The listing builds one solid part. Answer for the finished solid, in the listing's coordinates (mm). Face numbers are marked on the shaded views. A direction names the side the tool comes from. Coordinates: 2 decimals unless noted, no trailing zeros. Order: outer loops, then holes, each group sorted by start corner. A loop starts at its lowest first (then second) coordinate and runs counter-clockwise, first axis right, second up.
```python
from build123d import *

# Parameters (mm, degrees)
SKETCH1_W            = 68.5
SKETCH1_H            = 64.5
BOSS_EXTRUDE3_DEPTH  = 19
SKETCH3_W            = 60.5
SKETCH3_H            = 60.5
CUT_EXTRUDE1_DEPTH   = 15
SKETCH5_W            = 68.5
SKETCH5_H            = 4
BOSS_EXTRUDE4_DEPTH  = 105
SKETCH10_W           = 10
SKETCH10_H           = 29
BOSS_EXTRUDE5_DEPTH  = 5.5
SKETCH9_W            = 4
SKETCH9_H            = 20
CUT_EXTRUDE2_DEPTH   = 20.5
SKETCH11_W           = 6
SKETCH11_H           = 20
CUT_EXTRUDE3_DEPTH   = 5.5
CHAMFER2_SIZE        = 5.5
CHAMFER3_SIZE        = 2
SKETCH12_W           = 34.25
SKETCH12_H           = 169.5
CUT_EXTRUDE4_DEPTH   = 50
SKETCH15_R           = 1.5
CUT_EXTRUDE5_DEPTH   = 50
SKETCH16_R           = 1.5
CUT_EXTRUDE6_DEPTH   = 50
SKETCH17_R           = 1.5
CUT_EXTRUDE7_DEPTH   = 50
SKETCH19_W           = 34.25
SKETCH19_H           = 4
BOSS_EXTRUDE6_DEPTH  = 2
SKETCH26_W           = 4
SKETCH26_H           = 4
BOSS_EXTRUDE7_DEPTH  = 30
SKETCH20_R           = 3.75
CUT_EXTRUDE9_DEPTH   = 179.453250181
SKETCH21_W           = 3
SKETCH21_H           = 2.563068229
CUT_EXTRUDE10_DEPTH  = 5
SKETCH18_R           = 1.5
CUT_EXTRUDE8_DEPTH   = 135
SKETCH24_R           = 4
CUT_EXTRUDE13_DEPTH  = 178.441011325
SKETCH25_W           = 3
SKETCH25_H           = 2.291900756
CUT_EXTRUDE14_DEPTH  = 5
SKETCH27_R           = 1.75
CUT_EXTRUDE15_DEPTH  = 178.441011325
BOSS_EXTRUDE9_START  = 5
SKETCH30_W           = 8
SKETCH30_H           = 8
SKETCH30_R           = 1.75
BOSS_EXTRUDE9_DEPTH  = 5
SKETCH31_W           = 8
SKETCH31_H           = 8
CUT_EXTRUDE16_DEPTH  = 5
SKETCH32_W           = 19.705511252
SKETCH32_H           = 17.257631466
BOSS_EXTRUDE10_DEPTH = 5
SKETCH33_R           = 1.5
CUT_EXTRUDE17_DEPTH  = 5
SKETCH34_R           = 3.75
CUT_EXTRUDE18_DEPTH  = 5
SKETCH35_W           = 3
SKETCH35_H           = 2.563068229
CUT_EXTRUDE19_DEPTH  = 5


# Some blends are built 0.0001 mm under size
with BuildPart() as part:
    # Sketch1 → Boss-Extrude3 (new body)
    with BuildSketch(Plane(origin=(0, 0, 0), x_dir=(1, 0, 0), z_dir=(0, 1, 0))):
        with Locations((-34.25, 32.25)):
            Rectangle(SKETCH1_W, SKETCH1_H)
    extrude(amount=BOSS_EXTRUDE3_DEPTH)

    # Sketch3 → Cut-Extrude1 (cut)
    with BuildSketch(Plane(origin=(0, 19, 0), x_dir=(1, 0, 0), z_dir=(0, 1, 0))):
        with Locations((-34.25, 34.25)):
            Rectangle(SKETCH3_W, SKETCH3_H)
    extrude(amount=-CUT_EXTRUDE1_DEPTH, mode=Mode.SUBTRACT)

    # Sketch5 → Boss-Extrude4 (add)
    with BuildSketch(Plane(origin=(0, 0, -64.5), x_dir=(-1, 0, 0), z_dir=(0, 0, -1))):
        with Locations((34.25, 2)):
            Rectangle(SKETCH5_W, SKETCH5_H)
    extrude(amount=BOSS_EXTRUDE4_DEPTH)

    # Sketch10 → Boss-Extrude5 (add)
    with BuildSketch(Plane.XZ):
        with Locations((-5, -30)):
            Rectangle(SKETCH10_W, SKETCH10_H)
    extrude(amount=BOSS_EXTRUDE5_DEPTH)

    # Sketch9 → Cut-Extrude2 (cut)
    with BuildSketch(Plane(origin=(0, 19, 0), x_dir=(1, 0, 0), z_dir=(0, 1, 0))):
        with Locations((-2, 28)):
            Rectangle(SKETCH9_W, SKETCH9_H)
    extrude(amount=-CUT_EXTRUDE2_DEPTH, mode=Mode.SUBTRACT)

    # Sketch11 → Cut-Extrude3 (cut)
    with BuildSketch(Plane(origin=(0, 4, 0), x_dir=(1, 0, 0), z_dir=(0, 1, 0))):
        with Locations((-7, 28)):
            Rectangle(SKETCH11_W, SKETCH11_H)
    extrude(amount=-CUT_EXTRUDE3_DEPTH, mode=Mode.SUBTRACT)

    # Chamfer2
    chamfer2_edges = [part.edges().sort_by_distance(p)[0] for p in [
        (-5, -5.5, -44.5),
        (-5, -5.5, -15.5),
    ]]
    chamfer(chamfer2_edges, length=CHAMFER2_SIZE - 0.0001)  # a hair under: the kernel refuses the full size

    # Chamfer3
    # the kernel refuses this chamfer: 2 mm, written as the material it adds along each edge
    with BuildSketch(Plane(origin=(0, -1.5, -38), x_dir=(0, 0.9996219169112968, -0.027495876610585623), z_dir=(-1, 0, 0)), Plane(origin=(0, -1.5, -18), x_dir=(0, -0.027495876610586403, -0.9996219169112968), z_dir=(-1, 0, 0))) as chamfer3_piece_1:
        Polygon((CHAMFER3_SIZE * 0.999621916911, -CHAMFER3_SIZE * 0.0274958766106), (-CHAMFER3_SIZE * 0.0274958766106, -CHAMFER3_SIZE * 0.999621916911), (0, 0), align=None)
    extrude(amount=10)

    # Sketch12 → Cut-Extrude4 (cut)
    with BuildSketch(Plane(origin=(0, 19, 0), x_dir=(1, 0, 0), z_dir=(0, 1, 0))):
        with Locations((-51.375, 84.75)):
            Rectangle(SKETCH12_W, SKETCH12_H)
    extrude(amount=-CUT_EXTRUDE4_DEPTH, mode=Mode.SUBTRACT)

    # Sketch15 → Cut-Extrude5 (cut)
    with BuildSketch(Plane(origin=(0, -1.5, 0), x_dir=(1, 0, 0), z_dir=(0, 1, 0))):
        with Locations(Location((-5, 31.75713966, 0), (0, 0, 270))):
            Circle(SKETCH15_R)
    extrude(amount=-CUT_EXTRUDE5_DEPTH, mode=Mode.SUBTRACT)

    # Sketch16 → Cut-Extrude6 (cut)
    with BuildSketch(Plane(origin=(0, 4, 0), x_dir=(1, 0, 0), z_dir=(0, 1, 0))):
        with Locations(Location((-6, 6, 0), (0, 0, 270))):
            Circle(SKETCH16_R)
    extrude(amount=-CUT_EXTRUDE6_DEPTH, mode=Mode.SUBTRACT)

    # Sketch17 → Cut-Extrude7 (cut)
    with BuildSketch(Plane(origin=(0, 4, 0), x_dir=(1, 0, 0), z_dir=(0, 1, 0))):
        with Locations(Location((-6, 62.5, 0), (0, 0, 270))):
            Circle(SKETCH17_R)
    extrude(amount=-CUT_EXTRUDE7_DEPTH, mode=Mode.SUBTRACT)

    # Sketch19 → Boss-Extrude6 (add)
    with BuildSketch(Plane(origin=(0, 0, -169.5), x_dir=(-1, 0, 0), z_dir=(0, 0, -1))):
        with Locations((17.125, 2)):
            Rectangle(SKETCH19_W, SKETCH19_H)
    extrude(amount=BOSS_EXTRUDE6_DEPTH)

    # Sketch26 → Boss-Extrude7 (add)
    with BuildSketch(Plane(origin=(0, 4, 0), x_dir=(1, 0, 0), z_dir=(0, 1, 0))):
        with Locations((-2, 66.5)):
            Rectangle(SKETCH26_W, SKETCH26_H)
    extrude(amount=BOSS_EXTRUDE7_DEPTH)

    # Sketch20 → Cut-Extrude9 (cut, through all)
    with BuildSketch(Plane(origin=(0, -1.5, 0), x_dir=(1, 0, 0), z_dir=(0, 1, 0))):
        with Locations(Location((-5, 25.75713966, 0), (0, 0, 270))):
            Circle(SKETCH20_R)
    extrude(amount=-CUT_EXTRUDE9_DEPTH, mode=Mode.SUBTRACT)

    # Sketch21 → Cut-Extrude10 (cut)
    with BuildSketch(Plane(origin=(0, -1.5, 0), x_dir=(1, 0, 0), z_dir=(0, 1, 0))):
        with Locations((-5, 30.475605546)):
            Rectangle(SKETCH21_W, SKETCH21_H)
    extrude(amount=-CUT_EXTRUDE10_DEPTH, mode=Mode.SUBTRACT)

    # Sketch18 → Cut-Extrude8 (cut)
    with BuildSketch(Plane(origin=(0, 4, 0), x_dir=(1, 0, 0), z_dir=(0, 1, 0))):
        with Locations(Location((-13, 166.75713966, 0), (0, 0, 270))):
            Circle(SKETCH18_R)
    extrude(amount=-CUT_EXTRUDE8_DEPTH, mode=Mode.SUBTRACT)

    # Sketch24 → Cut-Extrude13 (cut, through all)
    with BuildSketch(Plane(origin=(0, 4, 0), x_dir=(1, 0, 0), z_dir=(0, 1, 0))):
        with Locations(Location((-13, 160.75713966, 0), (0, 0, 270))):
            Circle(SKETCH24_R)
    extrude(amount=-CUT_EXTRUDE13_DEPTH, mode=Mode.SUBTRACT)

    # Sketch25 → Cut-Extrude14 (cut)
    with BuildSketch(Plane(origin=(0, 4, 0), x_dir=(1, 0, 0), z_dir=(0, 1, 0))):
        with Locations((-13, 165.611189282)):
            Rectangle(SKETCH25_W, SKETCH25_H)
    extrude(amount=-CUT_EXTRUDE14_DEPTH, mode=Mode.SUBTRACT)

    # Sketch27 → Cut-Extrude15 (cut, through all)
    with BuildSketch(Plane(origin=(0, 4, 0), x_dir=(1, 0, 0), z_dir=(0, 1, 0))):
        with Locations(Location((-3, 72.5, 0), (0, 0, 270))):
            Circle(SKETCH27_R)
        with Locations(Location((-3, 158.5, 0), (0, 0, 270))):
            Circle(SKETCH27_R)
    extrude(amount=-CUT_EXTRUDE15_DEPTH, mode=Mode.SUBTRACT)

    # Sketch30 → Boss-Extrude9 (add)
    # profile 1 of 2: a face of its own
    with BuildSketch(Plane(origin=(0, 4, 0), x_dir=(1, 0, 0), z_dir=(0, 1, 0)).offset(BOSS_EXTRUDE9_START)):
        with Locations((-4, 72.5)):
            Rectangle(SKETCH30_W, SKETCH30_H)
        with Locations(Location((-3, 72.5, 0), (0, 0, 270))):
            Circle(SKETCH30_R, mode=Mode.SUBTRACT)
    # profile 2 of 2: a face of its own
    with BuildSketch(Plane(origin=(0, 4, 0), x_dir=(1, 0, 0), z_dir=(0, 1, 0)).offset(BOSS_EXTRUDE9_START)):
        with Locations((-4, 158.5)):
            Rectangle(SKETCH30_W, SKETCH30_H)
        with Locations(Location((-3, 158.5, 0), (0, 0, 270))):
            Circle(SKETCH30_R, mode=Mode.SUBTRACT)
    extrude(amount=-BOSS_EXTRUDE9_DEPTH)

    # Mirror5: part across plane


with BuildPart() as part_1:
    add(part.part)
    add(part.part.mirror(Plane(origin=(-34.25, 0, 0), x_dir=(0, 0, 1), z_dir=(1, 0, 0))))

    # Sketch31 → Cut-Extrude16 (cut)
    with BuildSketch(Plane(origin=(0, 9, 0), x_dir=(1, 0, 0), z_dir=(0, 1, 0))):
        with Locations((-64.5, 158.5)):
            Rectangle(SKETCH31_W, SKETCH31_H)
    extrude(amount=-CUT_EXTRUDE16_DEPTH, mode=Mode.SUBTRACT)

    # Sketch32 → Boss-Extrude10 (add)
    with BuildSketch(Plane(origin=(0, 4, 0), x_dir=(1, 0, 0), z_dir=(0, 1, 0))):
        with Locations((-58.647244374, 162.871184267)):
            Rectangle(SKETCH32_W, SKETCH32_H)
    extrude(amount=-BOSS_EXTRUDE10_DEPTH)

    # Sketch33 → Cut-Extrude17 (cut)
    with BuildSketch(Plane(origin=(0, 4, 0), x_dir=(1, 0, 0), z_dir=(0, 1, 0))):
        with Locations(Location((-62.5, 166.76, 0), (0, 0, 270))):
            Circle(SKETCH33_R)
    extrude(amount=-CUT_EXTRUDE17_DEPTH, mode=Mode.SUBTRACT)

    # Sketch34 → Cut-Extrude18 (cut)
    with BuildSketch(Plane(origin=(0, 4, 0), x_dir=(1, 0, 0), z_dir=(0, 1, 0))):
        with Locations(Location((-62.5, 160.76, 0), (0, 0, 270))):
            Circle(SKETCH34_R)
    extrude(amount=-CUT_EXTRUDE18_DEPTH, mode=Mode.SUBTRACT)

    # Sketch35 → Cut-Extrude19 (cut)
    with BuildSketch(Plane(origin=(0, 4, 0), x_dir=(1, 0, 0), z_dir=(0, 1, 0))):
        with Locations((-62.5, 165.478465886)):
            Rectangle(SKETCH35_W, SKETCH35_H)
    extrude(amount=-CUT_EXTRUDE19_DEPTH, mode=Mode.SUBTRACT)


solid = part_1.part
```
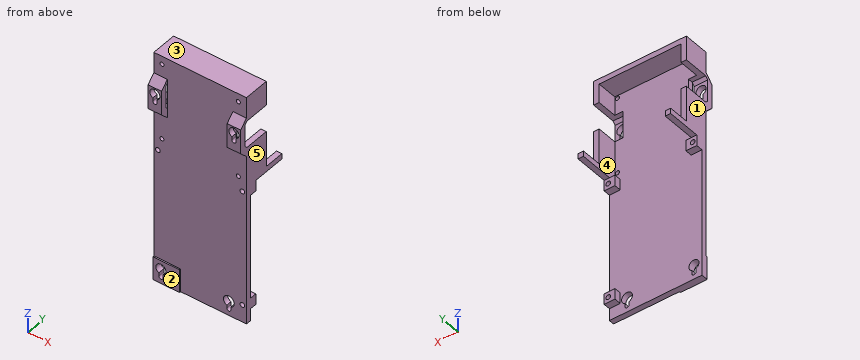
(1) Consider line 1 (X direction, y = 1.65, z = -6); line 2 (Z direction, x = -62.5, y = 2.55); line 3 (Z direction, x = -62, y = 1). Determine where each line is inside the solid, lowest interval first.
(2) Each of these flat-tipped pins is pushed along its axis until it touches: pin 1 Ø10 at (x, y) = (-10.5, 8.5) entering from +Z; pin 2 Ø4.5 at (x, y) = (-65.5, 29.5) entering from +Z; pin 3 Ø1.5 at (x, y) = (-4.5, 5.5) entering from -Z; pin 4 Ø8 at (x, y) = (-40.5, 9.5) entering from -Z. Where does it stop, or does it pass through?
(3) Find section B-B (z = -72.5). Write down the section's boundary in (x, y), and give its area (3 significant figures).
(4) For the marked faces 1 and 2, determine the directions among +Z, -Z, +X, -X, +Y, -Y from which every point of the face is accessible in a straight line to the end or side of a thin tool.
(5) Find section A-A (y = 21). Write down the section's boundary in (x, z), and give its area (3 significant figures).
(6) Find section C-C (y = 13). Write down the section's boundary in (x, z), and give its area (3 significant figures).
(7) The mould has two halves that part along Z. Classify the marked faces 3, 4 and 5: released by +Z, released by -Z, zero draft, split by the parting line, or undercut.
(8) Find section D-D (x = -54.5). Write down the section's boundary in (y, z).
Findings below:
1. line 1: x = -68.5 to -64, -61 to -7.5, -4.5 to 0
1. line 2: z = -171.5 to -168.26, -157.01 to -64, -61 to -38, -18 to -7.5, -4.5 to 0
1. line 3: z = -171.5 to -168.17, -157.04 to -63.91, -61.09 to -38, -18 to -7.41, -4.59 to 0
2. pin 1: stops at z = 0
2. pin 2: stops at z = -64.5
2. pin 3: stops at z = -162.5
2. pin 4: stops at z = -4
3. outline: (-68.5, 0) - (-67.25, 0) - (-67.25, 9) - (-68.5, 9) - close; (-63.75, 0) - (-4.75, 0) - (-4.75, 9) - (-8, 9) - (-8, 4) - (-60.5, 4) - (-60.5, 9) - (-63.75, 9) - close; (-1.25, 0) - (0, 0) - (0, 9) - (-1.25, 9) - close
3. area: 291 mm2
4. face 1: +Z, -Z, -X, +Y, -Y
4. face 2: -Z, +X, -X, -Y
5. outline: (-68.5, -68.5) - (-64.5, -68.5) - (-64.5, -64.5) - (-68.5, -64.5) - close; (-4, -68.5) - (0, -68.5) - (0, -64.5) - (-4, -64.5) - close
5. area: 32.0 mm2
6. outline: (-68.5, -68.5) - (-64.5, -68.5) - (-64.5, -38) - (-68.5, -38) - close; (-68.5, -18) - (-64.5, -18) - (-64.5, -4) - (-4, -4) - (-4, -18) - (0, -18) - (0, 0) - (-68.5, 0) - close; (-4, -68.5) - (0, -68.5) - (0, -38) - (-4, -38) - close
6. area: 630 mm2
7. face 3: released by +Z
7. face 4: undercut
7. face 5: zero draft
8. outline: (-1, -171.5) - (4, -171.5) - (4, -4) - (19, -4) - (19, 0) - (0, 0) - (0, -154.24) - (-1, -154.24) - close
